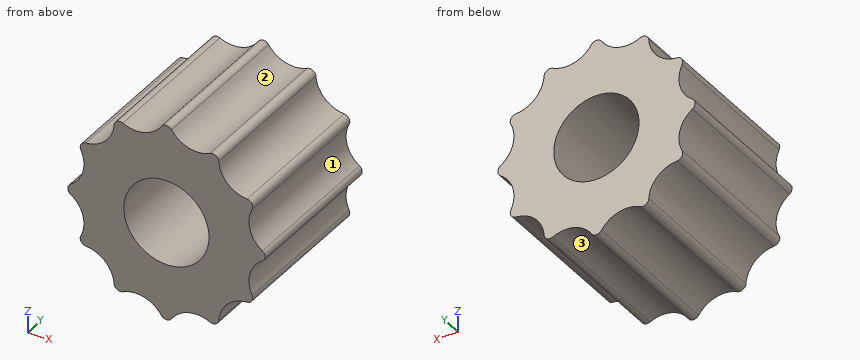
from build123d import *

# Parameters (mm, degrees)
SKETCH_1_R      = 2.1
EXTRUDE_1_DEPTH = 7.6
FILLET_1_R      = 0.3


with BuildPart() as part:
    # 草图1 → 凸台-拉伸1 (new body)
    with BuildSketch(Plane(origin=(0, 0, 0), x_dir=(1, 0, 0), z_dir=(0, 1, 0))):
        with BuildLine():
            ThreePointArc((-2.75, 4.763139721), (-1.102778373, 4.115624918), (0, 5.5))
            ThreePointArc((0, 5.5), (1.102778373, 4.115624918), (2.75, 4.763139721))
            ThreePointArc((2.75, 4.763139721), (3.012846545, 3.012846545), (4.763139721, 2.75))
            ThreePointArc((4.763139721, 2.75), (4.115624918, 1.102778373), (5.5, 0))
            ThreePointArc((5.5, 0), (4.115624918, -1.102778373), (4.763139721, -2.75))
            ThreePointArc((4.763139721, -2.75), (3.012846545, -3.012846545), (2.75, -4.763139721))
            ThreePointArc((2.75, -4.763139721), (1.102778373, -4.115624918), (0, -5.5))
            ThreePointArc((0, -5.5), (-1.102778373, -4.115624918), (-2.75, -4.763139721))
            ThreePointArc((-2.75, -4.763139721), (-3.012846545, -3.012846545), (-4.763139721, -2.75))
            ThreePointArc((-4.763139721, -2.75), (-4.115624918, -1.102778373), (-5.5, 0))
            ThreePointArc((-5.5, 0), (-4.115624918, 1.102778373), (-4.763139721, 2.75))
            ThreePointArc((-4.763139721, 2.75), (-3.012846545, 3.012846545), (-2.75, 4.763139721))
        make_face()
        Circle(SKETCH_1_R, mode=Mode.SUBTRACT)
    extrude(amount=EXTRUDE_1_DEPTH)

    # 圆角1
    fillet_1_edges = [part.edges().sort_by_distance(p)[0] for p in [
        (-2.75, 3.8, -4.763139721),
        (0, 3.8, -5.5),
        (2.75, 3.8, -4.763139721),
        (4.763139721, 3.8, -2.75),
        (5.5, 3.8, 0),
        (4.763139721, 3.8, 2.75),
        (2.75, 3.8, 4.763139721),
        (0, 3.8, 5.5),
        (-2.75, 3.8, 4.763139721),
        (-4.763139721, 3.8, 2.75),
        (-5.5, 3.8, 0),
        (-4.763139721, 3.8, -2.75),
    ]]
    fillet(fillet_1_edges, radius=FILLET_1_R)


solid = part.part
Could you check a few things on this model? Use its own coordinates, in mm. Face numbers are marked on the shaded views. Round coordinates to 2 decimals unless told otherwise and drop trailing zeros. Write each loop counter-clockwise with the first axis right and the second up, starting at its lowest first coordinate (ties: lowest second). Pieces come first, ordered by that corner, then holes. Notation, with made-up numbers: (46, 11.5) - (71, 11.5) arc R30 ccw to (71, 47.5) - close; hole circle Ø11 at (73, -13). An arc over 180 degrees is marked (long way). Put each result on its own line as item: value. Start each with the question number.
(1) I want a section at A-A, the plane z = -0.75. Please give me the cut outline in (x, y).
(2) I want a section at B-B, the plane x = -3. Please give me the cut outline in (y, z), plus the area to 3 significant figures.
(3) I need wall thicknesses on probe 1 along Z at (x, y) = (0, 5); probe 2 along Z at (x, y) = (4, 3.25). Which ranges of each line are inside material? Lowest first, please.
(4) Will this pin go through, and if not, where does the flat tip stop? pin 1 (2 mm diameter, centred on y = 2, z = -4, fed in from -X).
(5) I want a section at C-C, the plane z = 3.75. Please give me the cut outline in (x, y), plus the area to 3 significant figures.
(6) Thinking about a two-plate mould opening in Z: for the marked faces 1, 2 and 3, which applies, released by +Z, released by -Z, zero draft, split by the parting line, or undercut?
Here are the results:
1. outline: (-4.26, 0) - (-1.96, 0) - (-1.96, 7.6) - (-4.26, 7.6) - close; (1.96, 0) - (4.26, 0) - (4.26, 7.6) - (1.96, 7.6) - close
2. outline: (0, -3.03) - (7.6, -3.03) - (7.6, 3.03) - (0, 3.03) - close
2. area: 46.0 mm^2
3. probe 1: z = -4.86 to -2.1, 2.1 to 4.86
3. probe 2: z = -2.58 to 2.58
4. pin 1: stops at x = -3.03
5. outline: (-2.61, 0) - (2.61, 0) - (2.61, 7.6) - (-2.61, 7.6) - close
5. area: 39.7 mm^2
6. face 1: undercut
6. face 2: released by +Z
6. face 3: released by -Z
